Geometry: final body of the model. Coordinates: model frame, mm. Give positions to 0.01 mm unless a question says otherwise; leave off trailing zeros. Loops run counter-clockwise (first coordinate to the right, second up) from the corner with the lowest first, then second, coordinate; pieces in that order, holes last.
from build123d import *

# Parameters (mm, degrees)
SKETCH1_W               = 257.175
SKETCH1_H               = 257.175
BOSS_EXTRUDE1_DEPTH     = 3.175
SKETCH2_R               = 115.8875
CUT_EXTRUDE1_DEPTH      = 3.175
F_8_CLEARANCE_HOLE1_D   = 4.4958
FILLET1_R               = 12.7
F_3_8_CLEARANCE_HOLE1_D = 10.0838


with BuildPart() as part:
    # Sketch1 → Boss-Extrude1 (new body)
    with BuildSketch(Plane(origin=(0, 0, 0), x_dir=(1, 0, 0), z_dir=(0, 1, 0))):
        Rectangle(SKETCH1_W, SKETCH1_H)
    extrude(amount=BOSS_EXTRUDE1_DEPTH)

    # Sketch2 → Cut-Extrude1 (cut)
    with BuildSketch(Plane(origin=(0, 3.175, 0), x_dir=(1, 0, 0), z_dir=(0, 1, 0))):
        with Locations(Location((1.096399637, -1.096399637, 0), (0, 0, 270))):
            Circle(SKETCH2_R)
    extrude(amount=-CUT_EXTRUDE1_DEPTH, mode=Mode.SUBTRACT)

    # #8 Clearance Hole1 (through all)
    with Locations(Plane(origin=(0, 3.175, 0), x_dir=(1, 0, 0), z_dir=(0, 1, 0))):
        with Locations((87.000721301, -87.000721301), (123.0376, 0), (87.000721301, 87.000721301), (0, 123.0376), (-87.000721301, 87.000721301), (-123.0376, 0), (-87.000721301, -87.000721301), (0, -123.0376)):
            Hole(F_8_CLEARANCE_HOLE1_D / 2)

    # Fillet1
    fillet1_edges = [part.edges().sort_by_distance(p)[0] for p in [
        (128.5875, 1.5875, 128.5875),
        (-128.5875, 1.5875, 128.5875),
        (-128.5875, 1.5875, -128.5875),
        (128.5875, 1.5875, -128.5875),
    ]]
    fillet(fillet1_edges, radius=FILLET1_R)

    # 3/8 Clearance Hole1 (through all)
    with Locations(Plane(origin=(0, 3.175, 0), x_dir=(1, 0, 0), z_dir=(0, 1, 0))):
        with Locations((105.934238711, -105.934238711), (105.934238711, 105.934238711), (-105.934238711, -105.934238711), (-105.934238711, 105.934238711)):
            Hole(F_3_8_CLEARANCE_HOLE1_D / 2)


solid = part.part
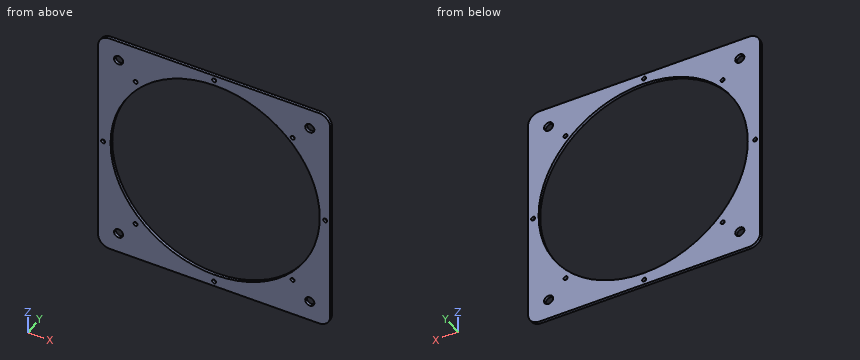
Item 1: Ray query, probe 1 along X at (y, z) = (1, 103.5); probe 2 along Z at (x, y) = (0, 1.8); probe 3 along Z at (x, y) = (105.5, 0.5). Return the intervals inside material, ascending.
Values follow:
probe 1: x = -128.59 to -110.35, -101.52 to -53.16, 55.35 to 101.52, 110.35 to 128.59
probe 2: z = -128.59 to -125.29, -120.79 to -114.79, 116.98 to 120.79, 125.29 to 128.59
probe 3: z = -128.59 to -110.96, -100.91 to -49.2, 51.39 to 100.91, 110.96 to 128.59
Item 2: Section query C-C on y = 1.9. Give the number of separate pieces and of enclosed holes in the cut face, plus the area to 3 significant figures.
Values follow:
separate pieces: 1
enclosed holes: 13
area: 23,400 mm2
Item 3: Section query D-D on x = -18. Return loops of the section in (y, z) (1 decimal).
Values follow:
outline: (0, -128.6) - (3.2, -128.6) - (3.2, -113.2) - (0, -113.2) - close; (0, 115.4) - (3.2, 115.4) - (3.2, 128.6) - (0, 128.6) - close
Item 4: Section query B-B on x = -104. Return loops of the section in (y, z) (1 decimal).
Values follow:
outline: (0, -128.6) - (3.2, -128.6) - (3.2, -110.6) - (0, -110.6) - close; (0, -101.3) - (3.2, -101.3) - (3.2, -47.7) - (0, -47.7) - close; (0, 49.9) - (3.2, 49.9) - (3.2, 101.3) - (0, 101.3) - close; (0, 110.6) - (3.2, 110.6) - (3.2, 128.6) - (0, 128.6) - close
Item 5: Section query A-A on z = -71. Return loops of the section in (x, y) (1 decimal).
Values follow:
outline: (-128.6, 0) - (-89.6, 0) - (-89.6, 3.2) - (-128.6, 3.2) - close; (91.8, 0) - (128.6, 0) - (128.6, 3.2) - (91.8, 3.2) - close
